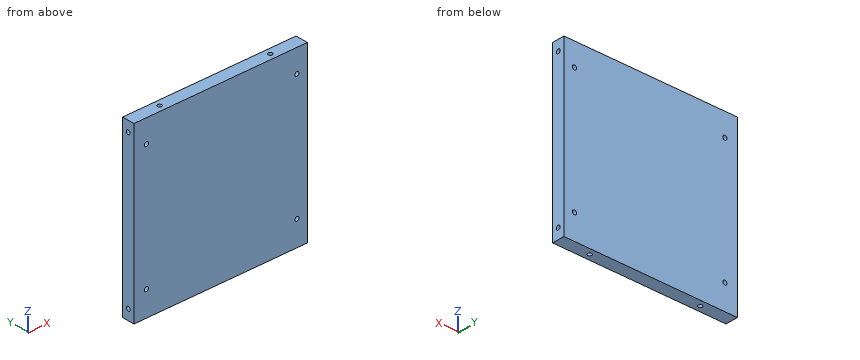
```python
from build123d import *

# Parameters (mm, degrees)
SKETCH1_W            = 83
SKETCH1_H            = 83
BOSS_EXTRUDE1_DEPTH  = 6
SKETCH2_R            = 1
CUT_EXTRUDE1_DEPTH   = 6
LPATTERN1_COUNT      = 2
LPATTERN1_PITCH      = 72
LPATTERN1_COUNT_DIR2 = 2
LPATTERN1_PITCH_DIR2 = 60
SKETCH3_R            = 1
CUT_EXTRUDE2_DEPTH   = 10
SKETCH4_R            = 1
CUT_EXTRUDE3_DEPTH   = 10


with BuildPart() as part:
    # Sketch1 → Boss-Extrude1 (new body)
    with BuildSketch(Plane(origin=(0, 0, 0), x_dir=(1, 0, 0), z_dir=(0, 1, 0))):
        with Locations((41.5, 41.5)):
            Rectangle(SKETCH1_W, SKETCH1_H)
    extrude(amount=BOSS_EXTRUDE1_DEPTH)

    # Sketch2 → Cut-Extrude1 (cut)
    with BuildSketch(Plane(origin=(0, 6, 0), x_dir=(1, 0, 0), z_dir=(0, 1, 0))):
        with Locations(Location((6, 71, 0), (0, 0, 270))):
            Circle(SKETCH2_R)
    cut_extrude1 = extrude(amount=-CUT_EXTRUDE1_DEPTH, mode=Mode.SUBTRACT)

    # LPattern1: Cut-Extrude1 2 × 2
    with Locations(*[(i * LPATTERN1_PITCH, 0, j * LPATTERN1_PITCH_DIR2) for i in range(LPATTERN1_COUNT) for j in range(LPATTERN1_COUNT_DIR2) if (i, j) != (0, 0)]):
        add(cut_extrude1, mode=Mode.SUBTRACT)

    # Sketch3 → Cut-Extrude2 (cut)
    with BuildSketch(Plane.ZY):
        with Locations((-78, 3)):
            Circle(SKETCH3_R)
        with Locations((-5, 3)):
            Circle(SKETCH3_R)
    cut_extrude2 = extrude(amount=-CUT_EXTRUDE2_DEPTH, mode=Mode.SUBTRACT)

    # Mirror1: Cut-Extrude2 across plane
    add(cut_extrude2.mirror(Plane.ZY.offset(-41.5)), mode=Mode.SUBTRACT)

    # Sketch4 → Cut-Extrude3 (cut)
    with BuildSketch(Plane.XY):
        with Locations((15, 3)):
            Circle(SKETCH4_R)
        with Locations((68, 3)):
            Circle(SKETCH4_R)
    cut_extrude3 = extrude(amount=-CUT_EXTRUDE3_DEPTH, mode=Mode.SUBTRACT)

    # Mirror2: Cut-Extrude3 across plane
    add(cut_extrude3.mirror(Plane.XY.offset(-41.5)), mode=Mode.SUBTRACT)


solid = part.part
```
Verification items for the finished model (mm, model axes). Give positions to 0.01 mm unless a question says otherwise; leave off trailing zeros. Loops run counter-clockwise (first coordinate to the right, second up) from the corner with the lowest first, then second, coordinate; pieces in that order, holes last. Notation, with made-up numbers: M 28,-39 L 38,-39 A20 ccw 38,-32 Z; hole C 77.5,10 d4. An arc over 180 degrees is marked long. One line per question, with ' | ' between items.
Item 1: Thickness scan on line 1 (X direction, y = 3.8, z = -71); line 2 (Y direction, x = 79.25, z = -78); line 3 (X direction, y = 2.8, z = -75.5). Record the ranges inside material, lowest first. Write a range as [from, to].
Completed:
line 1: x = [0, 5], [7, 77], [79, 83] | line 2: y = [0, 2], [4, 6] | line 3: x = [0, 14.02], [15.98, 67.02], [68.98, 83]
Item 2: Section check B-B, the plane z = -71. Record the cut outline in (x, y), plus the area to 3 significant figures.
Completed:
outline: M 0,0 L 5,0 L 5,6 L 0,6 Z; M 7,0 L 77,0 L 77,6 L 7,6 Z; M 79,0 L 83,0 L 83,6 L 79,6 Z | area: 474 mm^2
Item 3: Depth check by flat-ended pin: P1, Ø1.8, axis at x = 78, z = -11, coming from the +Y side; P2, Ø0.6, axis at y = 3, z = -5.5, coming from the -X side; P3, Ø1.8, axis at y = 3, z = -78, coming from the +X side. Enter the tip coordinate at first touch or a pass-through.
Completed:
P1: passes through | P2: stops at x = 10 | P3: stops at x = 73
Item 4: Section check A-A, the plane x = 78. Record the cut outline in (y, z), plus the area to 3 significant figures.
Completed:
outline: M 0,-83 L 6,-83 L 6,-72 L 0,-72 Z; M 0,-70 L 6,-70 L 6,-12 L 0,-12 Z; M 0,-10 L 6,-10 L 6,0 L 0,0 Z; hole C 3,-78 d2; hole C 3,-5 d2 | area: 468 mm^2
Item 5: Section check C-C, the plane z = -5. Record the cut outline in (x, y), plus the area to 3 significant figures.
Completed:
outline: M 0,0 L 83,0 L 83,2 L 73,2 L 73,4 L 83,4 L 83,6 L 0,6 L 0,4 L 10,4 L 10,2 L 0,2 Z; hole C 15,3 d2; hole C 68,3 d2 | area: 452 mm^2
Item 6: Section check D-D, the plane x = 68. Record the cut outline in (y, z).
Completed:
outline: M 0,-83 L 2,-83 L 2,-73 L 4,-73 L 4,-83 L 6,-83 L 6,0 L 4,0 L 4,-10 L 2,-10 L 2,0 L 0,0 Z
